from build123d import *

# Parameters (mm, degrees)
CROQUIS1_R              = 3
SALIENTE_EXTRUIR1_DEPTH = 10
CROQUIS2_R              = 3.25
SALIENTE_EXTRUIR2_DEPTH = 35
CROQUIS3_R              = 5
SALIENTE_EXTRUIR3_DEPTH = 17
CHAFL_N1_SIZE           = 2
CROQUIS4_R              = 1.25
SALIENTE_EXTRUIR4_DEPTH = 4


with BuildPart() as part:
    # Croquis1 → Saliente-Extruir1 (new body)
    with BuildSketch(Plane.XY):
        Circle(CROQUIS1_R)
    extrude(amount=SALIENTE_EXTRUIR1_DEPTH)

    # Croquis2 → Saliente-Extruir2 (add)
    with BuildSketch(Plane.XY.offset(10)):
        Circle(CROQUIS2_R)
    extrude(amount=SALIENTE_EXTRUIR2_DEPTH)

    # Croquis3 → Saliente-Extruir3 (add)
    with BuildSketch(Plane.XY.offset(45)):
        Circle(CROQUIS3_R)
    extrude(amount=SALIENTE_EXTRUIR3_DEPTH)

    # Chaflán1
    chafl_n1_edges = [part.edges().sort_by_distance(p)[0] for p in [
        (-5, 0, 62),
    ]]
    chamfer(chafl_n1_edges, length=CHAFL_N1_SIZE)

    # Croquis4 → Saliente-Extruir4 (add)
    with BuildSketch(Plane.XY.offset(62)):
        Circle(CROQUIS4_R)
    extrude(amount=SALIENTE_EXTRUIR4_DEPTH)


solid = part.part
For this review, take the finished solid that the model builds, in its own axes (mm). A direction names the side the tool comes from. Round coordinates to 2 decimals unless told otherwise and drop trailing zeros. Write each loop counter-clockwise with the first axis right and the second up, starting at its lowest first coordinate (ties: lowest second). Pieces come first, ordered by that corner, then holes. Notation, with made-up numbers: (65, -26.5) -> (91, -26.5) arc R20 ccw to (91, -11.5) -> close; hole circle Ø1 at (47.25, -3.75). An arc over 180 degrees is marked (long way). Use CSV: the item, a comma, the result in double quotes.
(1) Consider section D-D, the plane z = 49. Give the boundary of the cut face in (x, y), plus the area to 3 significant figures.
Computed values:
outline,"circle Ø10 at (0, 0)"
area,"78.5 mm²"
(2) Clearance check with flat-ended pins moving along their axes: P1, Ø4, axis at y = 1, z = 13, coming from the -X side; P2, Ø1, axis at x = -0.5, y = 3.5, coming from the -Z side; P3, Ø2, axis at y = -2.5, z = 36.5, coming from the +X side. State where each tip first meets the part, or that it passes through.
Computed values:
P1,"x = -3.25"
P2,"z = 10"
P3,"x = 2.88"
(3) For faces 1 (the face through (-1.08, -4.88, 52.4)), 2 (the face through (-0.27, -1.22, 63.97)), 3 (the face through (-3, 0, 5)), list the 3-axis set-ups (+Z, -Z, +X, -X, +Y, -Y) from which the entire face can be reached by the end or side of a thin tool; tool diameter is ignored.
Computed values:
face 1,"+Z, -Z"
face 2,"+Z"
face 3,"-Z"
(4) To check wall thickness, follow L1, parallel to Z at x = -1, y = -1.5; L2, parallel to X at y = -1.25, z = 35.5. State the ranges of each line that lie inside material, in increasing order. Write a range as [from, to].
Computed values:
L1,"[0, 62]"
L2,"[-3, 3]"
(5) Consider section C-C, the plane z = 29. Give the boundary of the cut face in (x, y), plus the area to 3 significant figures.
Computed values:
outline,"circle Ø6.5 at (0, 0)"
area,"33.2 mm²"
(6) Consider section A-A, the plane y = 0. Give the boundary of the cut face in (x, z).
Computed values:
outline,"(-5, 45) -> (-3.25, 45) -> (-3.25, 10) -> (-3, 10) -> (-3, 0) -> (3, 0) -> (3, 10) -> (3.25, 10) -> (3.25, 45) -> (5, 45) -> (5, 60) -> (3, 62) -> (1.25, 62) -> (1.25, 66) -> (-1.25, 66) -> (-1.25, 62) -> (-3, 62) -> (-5, 60) -> close"
